from build123d import *

# Parameters (mm, degrees)
BOSS_EXTRUDE1_DEPTH = 9.75
BOSS_EXTRUDE2_DEPTH = 2
SKETCH4_R           = 5.1
SKETCH4_R_2         = 3
SKETCH4_R_3         = 3.175
CUT_EXTRUDE1_DEPTH  = 55.534965848


with BuildPart() as part:
    # Sketch2 → Boss-Extrude1 (new, symmetric)
    with BuildSketch(Plane(origin=(0, 0, 0), x_dir=(0, 0, -1), z_dir=(1, 0, 0))):
        Polygon((-44, 0), (0, 0), (0, -20), (5, -20), (5, 30), (-44, 30), align=None)
    extrude(amount=BOSS_EXTRUDE1_DEPTH, both=True)

    # Sketch3 → Boss-Extrude2 (add)
    with BuildSketch(Plane(origin=(9.75, 0, 0), x_dir=(0, 0, -1), z_dir=(1, 0, 0))):
        Polygon((-44, 30), (-44, -4), (-15, -4), (-15, -20), (5, -20), (5, 30), align=None)
    boss_extrude2 = extrude(amount=BOSS_EXTRUDE2_DEPTH)

    # Mirror1: Boss-Extrude2 across plane
    add(boss_extrude2.mirror(Plane(origin=(0, 0, 0), x_dir=(0, 0, 1), z_dir=(1, 0, 0))))

    # Sketch4 → Cut-Extrude1 (cut, through all)
    with BuildSketch(Plane.XZ):
        with Locations(Location((0, 34, 0), (0, 0, 270))):
            Circle(SKETCH4_R)
        with Locations(Location((0, 19, 0), (0, 0, 270))):
            Circle(SKETCH4_R_2)
        with Locations(Location((0, 7, 0), (0, 0, 270))):
            Circle(SKETCH4_R_3)
    extrude(amount=-CUT_EXTRUDE1_DEPTH, mode=Mode.SUBTRACT)


solid = part.part
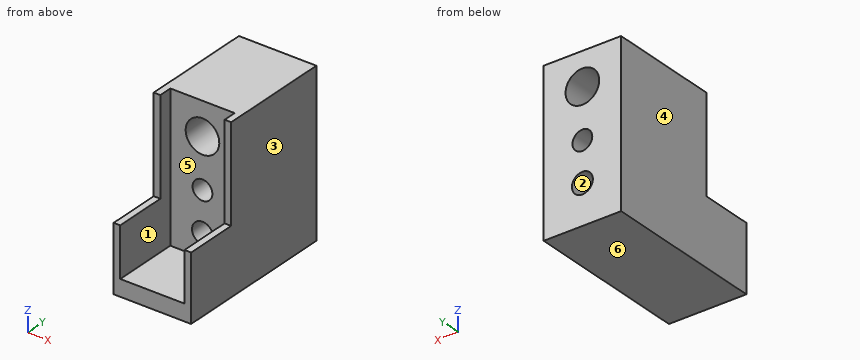
Check sheet for the modelled part. Datum: model origin and axes. Units: mm. Face numbers are marked on the shaded views. A direction names the side the tool comes from. Give positions to 0.01 mm unless a question says otherwise; leave off trailing zeros. Loops run counter-clockwise (first coordinate to the right, second up) from the corner with the lowest first, then second, coordinate; pieces in that order, holes last. Notation, with made-up numbers: M 2,72.5 L 49,72.5 A21 ccw 49,82.5 Z; hole C -33,-31 d8. An arc over 180 degrees is marked long. Return JSON: item names as keys, results as strings. Group by question number.
1. Tool access check on the marked faces 1 and 2. Record the directions out of +Z, -Z, +X, -X, +Y, -Y that give a thin tool (end or side, any length) a straight path to the whole face; none if there is none.
2. Cross-section at C-C on x = 0. Record the boundary of the cut face in (y, z) (3 decimals), plus the area to 4 significant figures.
3. Cross-section at A-A on y = 21. Record the boundary of the cut face in (x, z) (3 decimals), plus the area to 3 significant figures.
4. Cross-section at D-D on y = -6.5. Record the boundary of the cut face in (x, z), plus the area to 4 significant figures.
5. Mould release check, pull along X, two halves, no side actions. Record for the marked faces 3, 4, 5 and 6: released by +X, released by -X, zero draft, split by the parting line, or undercut.
6. Cross-section at B-B on z = 19. Record the boundary of the cut face in (x, y).
7. Thickness scan on L1, parallel to X at y = 18, z = 34; L2, parallel to X at y = 13.5, z = 19; L3, parallel to Z at x = -1.75, y = 24. Record the ranges inside material, lowest first.
8. Go/stop test with flat-tipped pins: pin 1 (2 mm diameter, centred on x = 10.5, z = 29, fed in from -Y); pin 2 (1.6 mm diameter, centred on x = -11, y = -11.5, fed in from +Z); pin 3 (10 mm diameter, centred on y = -13, z = 31, fed in from -X). Record where each tip stops, or that it passes through.
Return value:
{
 "1": {"face 1": "+Z, -Y", "face 2": "+Y, -Y"},
 "2": {"outline": "M -20,-5 L 30,-5 L 30,3.825 L 0,3.825 L 0,0 L -20,0 Z; M 0,10.175 L 30,10.175 L 30,16 L 0,16 Z; M 0,22 L 30,22 L 30,28.9 L 0,28.9 Z; M 0,39.1 L 30,39.1 L 30,44 L 0,44 Z", "area": "893.5 mm^2"},
 "3": {"outline": "M -11.75,-5 L 11.75,-5 L 11.75,44 L -11.75,44 Z; hole C 0,34 d10.2; hole C 0,7 d6.35; hole C 0,19 d6", "area": "1,010 mm^2"},
 "4": {"outline": "M -11.75,-5 L 11.75,-5 L 11.75,15 L 9.75,15 L 9.75,0 L -9.75,0 L -9.75,15 L -11.75,15 Z", "area": "177.5 mm^2"},
 "5": {"face 3": "released by +X", "face 4": "released by -X", "face 5": "undercut", "face 6": "zero draft"},
 "6": {"outline": "M -11.75,-4 L -9.75,-4 L -9.75,0 L -3,0 L -3,30 L -11.75,30 Z; M 3,0 L 9.75,0 L 9.75,-4 L 11.75,-4 L 11.75,30 L 3,30 Z"},
 "7": {"L1": "-11.75 to -5.1, 5.1 to 11.75", "L2": "-11.75 to -3, 3 to 11.75", "L3": "-5 to 4.35, 9.65 to 16.56, 21.44 to 29.21, 38.79 to 44"},
 "8": {"pin 1": "y = -4", "pin 2": "z = 15", "pin 3": "through"}
}
